```python
from build123d import *

# Parameters (mm, degrees)
SKETCH1_W           = 114.3
SKETCH1_H           = 139.7
BOSS_EXTRUDE1_DEPTH = 3.18
SKETCH2_R           = 1.5
SKETCH2_W           = 3.18
SKETCH2_H           = 59.975
CUT_EXTRUDE1_DEPTH  = 4.18
SKETCH3_W           = 3.18
SKETCH3_H           = 19.75
CUT_EXTRUDE2_DEPTH  = 3.18
SKETCH4_W           = 9.210739152
SKETCH4_H           = 39.093434174
CUT_EXTRUDE3_DEPTH  = 3.18


with BuildPart() as part:
    # Sketch1 → Boss-Extrude1 (new body)
    with BuildSketch(Plane.XY):
        Rectangle(SKETCH1_W, SKETCH1_H)
    extrude(amount=BOSS_EXTRUDE1_DEPTH)

    # Sketch2 → Cut-Extrude1 (cut, through all)
    with BuildSketch(Plane.XY.offset(3.18)):
        with Locations((-55.15, 0)):
            Circle(SKETCH2_R)
        with Locations((55.15, 0)):
            Circle(SKETCH2_R)
        Polygon((-10, 69.85), (10, 69.85), (10, 66.67), (1.5, 66.67), (1.5, 62.67), (3.5, 62.67), (3.5, 59.67), (1.5, 59.67), (1.5, 56.67), (-1.5, 56.67), (-1.5, 59.67), (-3.5, 59.67), (-3.5, 62.67), (-1.5, 62.67), (-1.5, 66.67), (-10, 66.67), align=None)
        Polygon((-10, -69.85), (-10, -66.67), (-1.5, -66.67), (-1.5, -62.67), (-3.5, -62.67), (-3.5, -59.67), (-1.5, -59.67), (-1.5, -56.67), (1.5, -56.67), (1.5, -59.67), (3.5, -59.67), (3.5, -62.67), (1.5, -62.67), (1.5, -66.67), (10, -66.67), (10, -69.85), align=None)
        with Locations((-55.56, 39.8625)):
            Rectangle(SKETCH2_W, SKETCH2_H)
        with Locations((-55.56, -39.8625)):
            Rectangle(SKETCH2_W, SKETCH2_H)
        with Locations((55.56, -39.8625)):
            Rectangle(SKETCH2_W, SKETCH2_H)
        with Locations((55.56, 39.8625)):
            Rectangle(SKETCH2_W, SKETCH2_H)
    extrude(amount=-CUT_EXTRUDE1_DEPTH, mode=Mode.SUBTRACT)

    # Sketch3 → Cut-Extrude2 (cut)
    with BuildSketch(Plane(origin=(0, 0, 0), x_dir=(-1, 0, 0), z_dir=(0, 0, -1))):
        with Locations((-17.401387583, 0)):
            Rectangle(SKETCH3_W, SKETCH3_H)
    extrude(amount=-CUT_EXTRUDE2_DEPTH, mode=Mode.SUBTRACT)

    # Sketch4 → Cut-Extrude3 (cut)
    with BuildSketch(Plane(origin=(0, 0, 0), x_dir=(-1, 0, 0), z_dir=(0, 0, -1))):
        with Locations((31.579688853, 0)):
            Rectangle(SKETCH4_W, SKETCH4_H)
    extrude(amount=-CUT_EXTRUDE3_DEPTH, mode=Mode.SUBTRACT)


solid = part.part
```
Source: CAD feature listing. Evaluate the final solid. Frame: model axes, mm. A direction names the side the tool comes from. Round coordinates to 2 decimals unless told otherwise and drop trailing zeros. Order: outer loops, then holes, each group sorted by start corner. A loop starts at its lowest first (then second) coordinate and runs counter-clockwise, first axis right, second up. Notation, with made-up numbers: (-0.75, -14.5) -> (11.25, -14.5) arc R12 ccw to (11.25, 8.5) -> close; hole circle Ø9 at (53.25, -20.75). An arc over 180 degrees is marked (long way). Use CSV: the item, a comma, the result in double quotes.
(1) Section B-B on z = 1.45. Count the separate pieces of the cut face and the enclosed holes in it, and give its area (3 significant figures).
Report:
separate pieces,"1"
enclosed holes,"4"
area,"14,600 mm^2"
(2) Pull-direction query (Y, two-part tool) for faces 1 (the face through (0, -56.67, 2)), 2 (the face through (57.15, 0, 2)), 3 (the face through (-3.5, 61, 2)); classes: +Y half, -Y half, draft (parallel to the pull), parting line (faces both ways), or undercut.
Report:
face 1,"-Y half"
face 2,"draft"
face 3,"undercut"
(3) Section A-A on y = 0. Return the cut outline in (x, z).
Report:
outline,"(-57.15, 0) -> (-56.65, 0) -> (-56.65, 3.18) -> (-57.15, 3.18) -> close; (-53.65, 0) -> (-36.19, 0) -> (-36.19, 3.18) -> (-53.65, 3.18) -> close; (-26.97, 0) -> (15.81, 0) -> (15.81, 3.18) -> (-26.97, 3.18) -> close; (18.99, 0) -> (53.65, 0) -> (53.65, 3.18) -> (18.99, 3.18) -> close; (56.65, 0) -> (57.15, 0) -> (57.15, 3.18) -> (56.65, 3.18) -> close"
(4) Access query for faces 4 (the face through (-1.5, -58, 2)), 5 (the face through (53.97, -40, 2)), 6 (the face through (-32, -19.547, 2)), 7 (the face through (-53.97, 39, 2)), 8 (the face through (-56, -9.875, 2)). Directions: +Z, -Z, +X, -X, +Y, -Y. A direction counts if a zero-diameter tool reaches every point of the face in a straight line with its end or side. Return the directions, or none.
Report:
face 4,"+Z, -Z, -Y"
face 5,"+Z, -Z, +X, -Y"
face 6,"+Z, -Z"
face 7,"+Z, -Z, -X, +Y"
face 8,"+Z, -Z, -X, -Y"
(5) Ray query, L1, parallel to Y at x = 55.15, z = 2.45 (3 decimals); L2, parallel to X at y = -62, z = 2.2; L3, parallel to X at y = -31.5, z = 1.3. Return the intervals inside material, ascending.
Report:
L1,"-9.875 to -1.5, 1.5 to 9.875"
L2,"-53.97 to -3.5, 3.5 to 53.97"
L3,"-53.97 to 53.97"
(6) Section C-C on x = -6.5. Return the cut outline in (y, z).
Report:
outline,"(-66.67, 0) -> (66.67, 0) -> (66.67, 3.18) -> (-66.67, 3.18) -> close"
(7) Section D-D on y = 25. Return the cut outline in (x, z), and give its area (3 significant figures).
Report:
outline,"(-53.97, 0) -> (53.97, 0) -> (53.97, 3.18) -> (-53.97, 3.18) -> close"
area,"343 mm^2"
(8) First-contact query: pin 1 Ø1.6 at (y, z) = (68, 2) entering from +X; pin 2 Ø0.9 at (y, z) = (58, 2) entering from -X; pin 3 Ø1 at (x, z) = (2.5, 2) entering from +Y. Flat tips, straight axial feed; report the tip coordinate or a pass-through.
Report:
pin 1,"x = 53.97"
pin 2,"x = -53.97"
pin 3,"y = 66.67"
